Answer from the drawing. Dimensions are ordinates in mm from the lowest x, y and z of the part. A direction names the side the tool comes from. Round coordinates to 2 decimals unless told otherwise and drop trailing zeros. Loops run counter-clockwise (first coordinate to the right, second up) from the corner with the lowest first, then second, coordinate; pieces in that order, holes last. Notation, with made-up numbers: (27, -6.5) - (31, -6.5) arc R18 cw to (31, 1.5) - close; hole circle Ø11 at (20.25, 51). An arc over 180 degrees is marked (long way). Return JSON: item names as keys, results as strings.
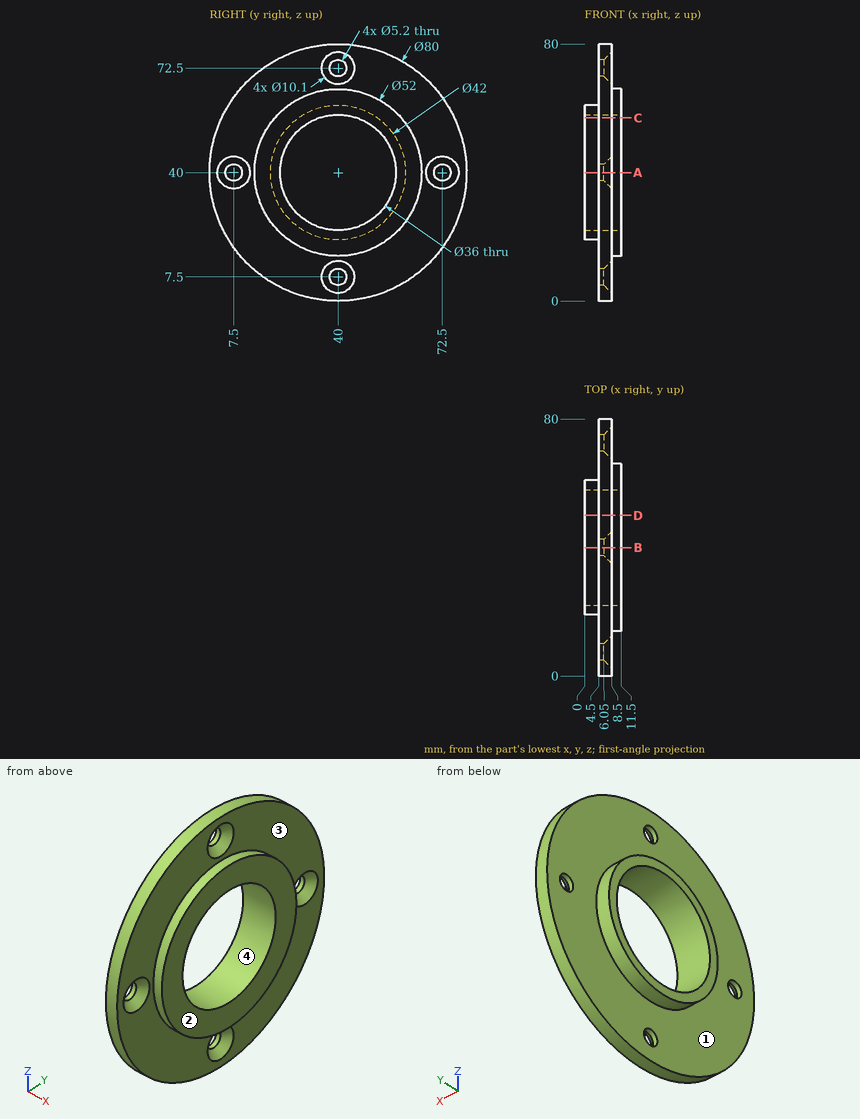
1) Determine the mould class of the marked faces 3 and 4 for opening direction Y: pulls with the +Y half, pulls with the -Y half, needs draft (parallel to the pull), parting line crosses it, or undercut.
Verdict:
{"face 3": "needs draft", "face 4": "undercut"}
2) Find the intervals of material crossed by L1, parallel to Y at x = 5.6, z = 40; L2, parallel to Y at x = 6.25, z = 42; L3, parallel to X at y = 51, z = 6, in increasing order.
Verdict:
{"L1": "y = 0 to 4.9, 10.1 to 22, 58 to 69.9, 75.1 to 80", "L2": "y = 0.05 to 5.54, 9.46 to 22.11, 57.89 to 70.54, 74.46 to 79.95", "L3": "x = 4.5 to 8.5"}
3) Section A-A (z = 40) is taken. Give the vertices of the cut face in (x, y).
Verdict:
{"outline": "(0, 19) - (4.5, 19) - (4.5, 10.1) - (6.05, 10.1) - (8.5, 12.55) - (8.5, 14) - (11.5, 14) - (11.5, 22) - (0, 22) - close; (0, 58) - (11.5, 58) - (11.5, 66) - (8.5, 66) - (8.5, 67.45) - (6.05, 69.9) - (4.5, 69.9) - (4.5, 61) - (0, 61) - close; (4.5, 0) - (8.5, 0) - (8.5, 2.45) - (6.05, 4.9) - (4.5, 4.9) - close; (4.5, 75.1) - (6.05, 75.1) - (8.5, 77.55) - (8.5, 80) - (4.5, 80) - close"}
4) Section C-C (z = 57) is taken. Give the vertices of the cut face in (x, y).
Verdict:
{"outline": "(0, 27.67) - (4.5, 27.67) - (4.5, 3.79) - (8.5, 3.79) - (8.5, 20.33) - (11.5, 20.33) - (11.5, 34.08) - (0, 34.08) - close; (0, 45.92) - (11.5, 45.92) - (11.5, 59.67) - (8.5, 59.67) - (8.5, 76.21) - (4.5, 76.21) - (4.5, 52.33) - (0, 52.33) - close"}
5) A tool of negligible diameter and unlimited length cuts with its end or side. For the marked faces 1 and 2, from which of +Z, -Z, +X, -X, +Y, -Y can it reach the whole face along a straight path? Write none if from no direction.
Verdict:
{"face 1": "-X", "face 2": "+Z, -Z, +X, +Y, -Y"}
6) Flat-ended cylindrical pins translate along their axes: pin 1 (1 mm diameter, centred on x = 4.5, z = 58.5, fed in from -Y); pin 2 (1.5 mm diameter, centred on x = 7, y = 69, fed in from -Z); pin 3 (21.5 mm diameter, centred on y = 40, z = 40, fed in from +X); pin 4 (1 mm diameter, centred on x = 6, y = 33.5, fed in from +Z). Find the tip coordinate at first contact, or state that the pin passes through.
Verdict:
{"pin 1": "stops at y = 4.28", "pin 2": "stops at z = 11.68", "pin 3": "passes through", "pin 4": "stops at z = 79.55"}
7) Section D-D (y = 50) is taken. Give the vertices of the cut face in (x, z).
Verdict:
{"outline": "(0, 21.53) - (4.5, 21.53) - (4.5, 1.27) - (8.5, 1.27) - (8.5, 16) - (11.5, 16) - (11.5, 25.03) - (0, 25.03) - close; (0, 54.97) - (11.5, 54.97) - (11.5, 64) - (8.5, 64) - (8.5, 78.73) - (4.5, 78.73) - (4.5, 58.47) - (0, 58.47) - close"}
